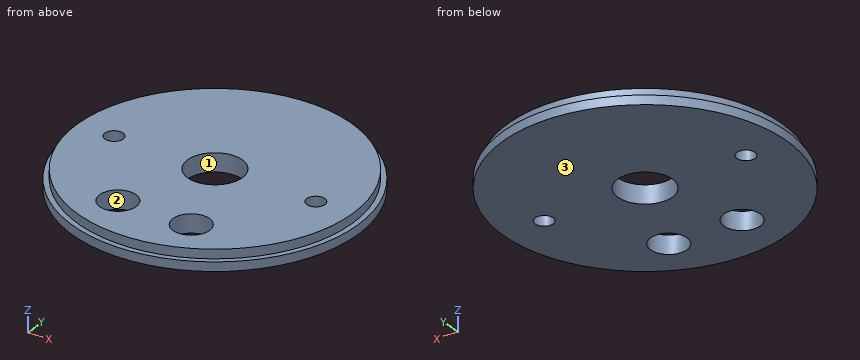
```python
from build123d import *

# Parameters (mm, degrees)
SKETCH1_R           = 49.5046
BOSS_EXTRUDE1_DEPTH = 3.175
SKETCH2_R           = 47.6885
BOSS_EXTRUDE2_DEPTH = 3.175
SKETCH3_R           = 6.35
SKETCH3_R_2         = 3.175
SKETCH3_R_3         = 9.525
CUT_EXTRUDE1_DEPTH  = 71.297463271


with BuildPart() as part:
    # Sketch1 → Boss-Extrude1 (new body)
    with BuildSketch(Plane.XY):
        Circle(SKETCH1_R)
    extrude(amount=BOSS_EXTRUDE1_DEPTH)

    # Sketch2 → Boss-Extrude2 (add)
    with BuildSketch(Plane.XY.offset(3.175)):
        Circle(SKETCH2_R)
    extrude(amount=BOSS_EXTRUDE2_DEPTH)

    # Sketch3 → Cut-Extrude1 (cut, through all)
    with BuildSketch(Plane.XY.offset(6.35)):
        with Locations((-12.7, -31.235352443)):
            Circle(SKETCH3_R)
        with Locations((12.7, -31.235352443)):
            Circle(SKETCH3_R)
        with Locations((-34.925, 0)):
            Circle(SKETCH3_R_2)
        with Locations((34.925, 0)):
            Circle(SKETCH3_R_2)
        Circle(SKETCH3_R_3)
    extrude(amount=-CUT_EXTRUDE1_DEPTH, mode=Mode.SUBTRACT)


solid = part.part
```
The model under review builds one solid part; all positions refer to its coordinate system, in mm. Face numbers are marked on the shaded views. Give positions to 0.01 mm unless a question says otherwise; leave off trailing zeros. Write each loop counter-clockwise with the first axis right and the second up, starting at its lowest first coordinate (ties: lowest second). Pieces come first, ordered by that corner, then holes. Notation, with made-up numbers: (41, -31) -> (81, -31) arc R38 ccw to (81, 7) -> close; hole circle Ø8 at (54.5, 5.25). An arc over 180 degrees is marked (long way). Put each result on its own line as item: value.
(1) We need section C-C, the plane z = 1. Give the boundary of the cut face in (x, y) (3 decimals), and give its area (3 significant figures).
Results are:
outline: circle Ø99.009 at (0, 0); hole circle Ø6.35 at (-34.925, 0); hole circle Ø12.7 at (-12.7, -31.235); hole circle Ø19.05 at (0, 0); hole circle Ø12.7 at (12.7, -31.235); hole circle Ø6.35 at (34.925, 0)
area: 7,100 mm²
(2) To check wall thickness, follow probe 1 along Y at (x, z) = (0, 2.75) (3 decimals); probe 2 along Y at (x, z) = (7.5, 3.5); probe 3 along X at (y, z) = (-36, 3). State the ranges of each line that lie inside material, in increasing order. Write a range as from..to.
Results are:
probe 1: -49.505..-9.525, 9.525..49.505
probe 2: -47.1..-34.88, -27.59..-5.87, 5.87..47.1
probe 3: -33.98..-16.9, -8.5..8.5, 16.9..33.98
(3) We need section A-A, the plane y = 0. State how many separate pieces and enclosed holes the cut face has, and give its area (3 significant figures).
Results are:
separate pieces: 4
enclosed holes: 0
area: 416 mm²
(4) The part is to be moulded in two halves that separate along X. For the marked faces 1, 2 and 3, say which applies: pulls with the +X half, pulls with the -X half, needs draft (parallel to the pull), parting line crosses it, or undercut.
Results are:
face 1: undercut
face 2: undercut
face 3: needs draft
(5) For pin 1 Ø5.5 at (x, y) = (34.925, 0) entering from +Z, flat-tipped, find the tip position at first contact; note if it passes through.
Results are:
pin 1: through
(6) We need section D-D, the plane x = -12.7. Give the boundary of the cut face in (y, z) (3 decimals), and give its area (3 significant figures).
Results are:
outline: (-47.848, 0) -> (-37.585, 0) -> (-37.585, 6.35) -> (-45.966, 6.35) -> (-45.966, 3.175) -> (-47.848, 3.175) -> close; (-24.885, 0) -> (47.848, 0) -> (47.848, 3.175) -> (45.966, 3.175) -> (45.966, 6.35) -> (-24.885, 6.35) -> close
area: 515 mm²
